For this review, take the finished solid that the model builds, in its own axes (mm). Coordinates: 2 decimals unless noted, no trailing zeros. Order: outer loops, then holes, each group sorted by start corner. A loop starts at its lowest first (then second) coordinate and runs counter-clockwise, first axis right, second up. Notation, with made-up numbers: M 88.25,0 L 103.25,0 A29 cw 103.25,25 Z; hole C 30.25,45.5 d1. An arc over 180 degrees is marked long. Use CSV: the item, a comma, the result in double quotes.
```python
from build123d import *

# Parameters (mm, degrees)
ESQUISSE1_R        = 3
ESQUISSE1_R_2      = 0.75
BOSS_EXTRU_1_DEPTH = 12
CHANFREIN1_SIZE    = 3
CHANFREIN1_SIZE2   = 1
CHANFREIN2_SIZE    = 1
CHANFREIN2_SIZE2   = 3


with BuildPart() as part:
    # Esquisse1 → Boss.-Extru.1 (new body)
    with BuildSketch(Plane.XY):
        Circle(ESQUISSE1_R)
        Circle(ESQUISSE1_R_2, mode=Mode.SUBTRACT)
    extrude(amount=BOSS_EXTRU_1_DEPTH)

    # Chanfrein1
    chanfrein1_edges = [part.edges().sort_by_distance(p)[0] for p in [
        (-3, 0, 12),
    ]]
    chanfrein1_side = [part.faces().sort_by_distance(p)[0] for p in [
        (-3, 0, 6),
    ]]
    chamfer(chanfrein1_edges, length=CHANFREIN1_SIZE, length2=CHANFREIN1_SIZE2, reference=chanfrein1_side[0])

    # Chanfrein2
    chanfrein2_edges = [part.edges().sort_by_distance(p)[0] for p in [
        (-3, 0, 0),
    ]]
    chanfrein2_side = [part.faces().sort_by_distance(p)[0] for p in [
        (-2.915147186, 0, 0),
    ]]
    chamfer(chanfrein2_edges, length=CHANFREIN2_SIZE, length2=CHANFREIN2_SIZE2, reference=chanfrein2_side[0])


solid = part.part
```
Item 1: To check wall thickness, follow line 1 along Y through (x, z) = (0, 9); line 2 along X through (y, z) = (0.35, 6); line 3 along Y through (x, z) = (0, 2.5). State the ranges of each line that lie inside material, in increasing order. Write a range as [from, to].
Solutions:
line 1,"[-3, -0.75], [0.75, 3]"
line 2,"[-2.98, -0.66], [0.66, 2.98]"
line 3,"[-2.83, -0.75], [0.75, 2.83]"
Item 2: Draft analysis for pull direction X (two halves, no side actions). For faces 1 (the face through (-3, 0, 6)), 2 (the face through (1, 0, 12)), 3 (the face through (-0.75, 0.03, 5.92)), state which applies: released by +X, released by -X, zero draft, split by the parting line, or undercut.
Solutions:
face 1,"split by the parting line"
face 2,"zero draft"
face 3,"undercut"
Item 3: Add section C-C on z = 6. State the section outline as (x, y) points, and give its area (3 significant figures).
Solutions:
outline,"C 0,0 d6; hole C 0,0 d1.5"
area,"26.5 mm^2"
Item 4: Clearance check with flat-ended pins moving along their axes: pin 1 Ø1 at (y, z) = (1.5, 6.5) entering from +X; pin 2 Ø0.9 at (x, y) = (0, 0) entering from -Z. State where each tip first meets the part, or that it passes through.
Solutions:
pin 1,"x = 2.83"
pin 2,"through"
Item 5: Add section D-D on z = 2.5. State the section outline as (x, y) points.
Solutions:
outline,"C 0,0 d5.67; hole C 0,0 d1.5"
Item 6: Add section A-A on y = 0. State the section outline as (x, z) points.
Solutions:
outline,"M -3,3 L -2,0 L -0.75,0 L -0.75,12 L -2,12 L -3,9 Z; M 0.75,0 L 2,0 L 3,3 L 3,9 L 2,12 L 0.75,12 Z"
